Design review of the part built by this model. Coordinates are the model's own, in mm. Round coordinates to 2 decimals unless told otherwise and drop trailing zeros. Loops run counter-clockwise (first coordinate to the right, second up) from the corner with the lowest first, then second, coordinate; pieces in that order, holes last. Notation, with made-up numbers: M 89,9 L 134,9 A13 cw 134,27 Z; hole C -10.75,82 d8. An arc over 180 degrees is marked long. One line per item, written item: value. Start each with the question number.
Item 1: For line 1 along Y through (x, z) = (-12, 6.75), list the stretches that pass through material, from the lowest coordinate up.
Item 2: We need section C-C (z = 4.25). Write out the cut boundary in (x, y), then the cut area to 3 significant figures.
Item 3: We need section B-B (x = -0.75). Write out the cut boundary in (y, z).
Item 4: We need section A-A (z = 3). Write out the cut boundary in (x, y), then the cut area to 3 significant figures.
from build123d import *

# Parameters (mm, degrees)
SKETCH_1_W      = 28
SKETCH_1_H      = 15
EXTRUDE_1_DEPTH = 11
SKETCH_2_R      = 0.5
EXTRUDE_2_DEPTH = 2


with BuildPart() as part:
    # 草图1 → 凸台-拉伸1 (new body)
    with BuildSketch(Plane.XY):
        Rectangle(SKETCH_1_W, SKETCH_1_H)
    extrude(amount=EXTRUDE_1_DEPTH)

    # 草图2 → 凸台-拉伸2 (add)
    with BuildSketch(Plane(origin=(0, 7.5, 0), x_dir=(1, 0, 0), z_dir=(0, 1, 0))):
        with Locations(Location((-11.594640153, -2.971812887, 0), (0, 0, 90))):
            Circle(SKETCH_2_R)
        with Locations(Location((-11.594640153, -8.028187113, 0), (0, 0, 90))):
            Circle(SKETCH_2_R)
    extrude(amount=EXTRUDE_2_DEPTH)


solid = part.part
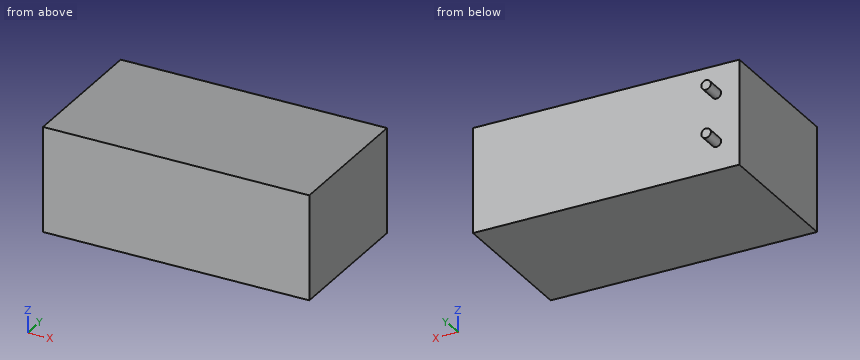
A:
1. line 1: -7.5 to 7.5
2. outline: M -14,-7.5 L 14,-7.5 L 14,7.5 L -14,7.5 Z
2. area: 420 mm2
3. outline: M -7.5,0 L 7.5,0 L 7.5,11 L -7.5,11 Z
4. outline: M -14,-7.5 L 14,-7.5 L 14,7.5 L -11.1,7.5 L -11.1,9.5 L -12.09,9.5 L -12.09,7.5 L -14,7.5 Z
4. area: 422 mm2
